Build history of the part. All positions in model axes, mm. Face numbers are marked on the shaded views. A direction names the side the tool comes from. Round coordinates to 2 decimals unless told otherwise and drop trailing zeros. Write each loop counter-clockwise with the first axis right and the second up, starting at its lowest first coordinate (ties: lowest second). Pieces come first, ordered by that corner, then holes. Notation, with made-up numbers: M 86,59 L 124,59 A18 ccw 124,88 Z; hole C 84.5,59.25 d6. An arc over 180 degrees is marked long. Use a Markdown table: item, result.
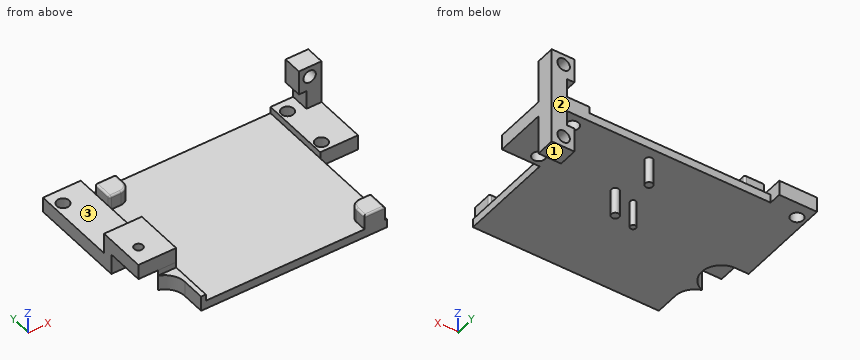
from build123d import *

# Parameters (mm, degrees)
CYLINDER022_R     = 1.15
CYLINDER022_DEPTH = 10
EXTRUDE025_DEPTH  = 1.5
SKETCH022_R       = 0.75
SKETCH022_R_2     = 1
EXTRUDE022_DEPTH  = 8
BOX005_W          = 48
BOX005_H          = 45
BOX005_DEPTH      = 10
SKETCH020_R       = 1.65
EXTRUDE020_DEPTH  = 4
EXTRUDE001_DEPTH  = 4
FILLET003_R       = 0.5
SKETCH021_R       = 1.65
EXTRUDE021_DEPTH  = 5
BOX006_W          = 10
BOX006_H          = 12.95
BOX006_DEPTH      = 4


with BuildPart() as cylinder022:
    # Cylinder022 → Cylinder022 (new body)
    with BuildSketch(Plane(origin=(6.5, 51, 13.03), x_dir=(1, 0, 0), z_dir=(0, 0, 1))):
        Circle(CYLINDER022_R)
    extrude(amount=CYLINDER022_DEPTH)


with BuildPart() as extrude025:
    # Sketch028 → Extrude025 (new body)
    with BuildSketch(Plane.XY):
        with BuildLine():
            Line((8.25, 46.050253), (13, 46.050253))
            Line((13, 46.050253), (13, 59))
            Line((13, 59), (3, 59))
            Line((3, 59), (3, 56.25))
            Line((3, 56.25), (6.5, 56.25))
            ThreePointArc((8.25, 46.050253), (11.674392, 51.887785), (6.5, 56.25))
        make_face()
    extrude(amount=EXTRUDE025_DEPTH)


with BuildPart() as extrude025_1:
    # Extrude025 placement: moved
    add(extrude025.part.moved(Location((0, 0, 17))))


with BuildPart() as extrude022:
    # Sketch022 → Extrude022 (new body)
    with BuildSketch(Plane.XY):
        with Locations((37.45, 61.7)):
            Circle(SKETCH022_R)
        with Locations((42.85, 62.65)):
            Circle(SKETCH022_R_2)
        with Locations((42.85, 75.35)):
            Circle(SKETCH022_R_2)
    extrude(amount=EXTRUDE022_DEPTH)


with BuildPart() as extrude022_1:
    # Extrude022 placement: moved
    add(extrude022.part.moved(Location((0, 0, 6))))


with BuildPart() as obj1:
    # Box005 → Box005 (new body)
    with BuildSketch(Plane(origin=(13, 34, 15.25), x_dir=(1, 0, 0), z_dir=(0, 0, 1))):
        with Locations((24, 22.5)):
            Rectangle(BOX005_W, BOX005_H)
    extrude(amount=BOX005_DEPTH)


with BuildPart() as sensorhold:
    # Sketch020 → Extrude020 (new body)
    with BuildSketch(Plane.XY):
        with BuildLine():
            Line((3, 56.25), (3, 82))
            Line((3, 82), (13, 82))
            Line((13, 82), (13, 78.75))
            Line((13, 78.75), (71, 78.75))
            Line((71, 78.75), (71, 60))
            Line((61, 60), (71, 60))
            Line((61, 34.86), (61, 60))
            Line((11.75, 34.86), (61, 34.86))
            Line((11.75, 34.86), (11.75, 41))
            ThreePointArc((11.75, 41), (10.740672, 44.095028), (8.100781, 46))
            ThreePointArc((8.100781, 46), (11.687123, 51.810093), (6.5, 56.25))
            Line((3, 56.25), (6.5, 56.25))
        make_face()
        with Locations((5.45, 77.95)):
            Circle(SKETCH020_R, mode=Mode.SUBTRACT)
        with Locations((63.15, 62.65)):
            Circle(SKETCH020_R, mode=Mode.SUBTRACT)
        with Locations((63.15, 75.4)):
            Circle(SKETCH020_R, mode=Mode.SUBTRACT)
    extrude(amount=EXTRUDE020_DEPTH)


with BuildPart() as sensorhold_1:
    # Extrude020 placement: moved
    add(sensorhold.part.moved(Location((0, 0, 13))))

    # Cut007: cut obj1
    add(obj1.part, mode=Mode.SUBTRACT)


with BuildPart() as obj2:
    # Sketch001 → Extrude001 (new body)
    with BuildSketch(Plane.XY):
        with BuildLine():
            Line((19.03, 74.44), (19.03, 77.44))
            Line((19.03, 77.44), (13.53, 77.44))
            Line((13.53, 71.94), (13.53, 77.44))
            Line((16.53, 71.94), (13.53, 71.94))
            ThreePointArc((16.53, 71.94), (18.297767, 72.672233), (19.03, 74.44))
        make_face()
        with BuildLine():
            Line((60.53, 34.86), (55.03, 34.86))
            Line((55.03, 34.86), (55.03, 37.86))
            ThreePointArc((57.53, 40.36), (55.762233, 39.627767), (55.03, 37.86))
            Line((60.53, 40.36), (57.53, 40.36))
            Line((60.53, 34.86), (60.53, 40.36))
        make_face()
    extrude(amount=EXTRUDE001_DEPTH)


with BuildPart() as obj2_1:
    # Extrude001 placement: moved
    add(obj2.part.moved(Location((0, 0, 2))))

    # Fillet003
    fillet003_edges = [obj2_1.edges().sort_by_distance(p)[0] for p in [
        (57.78, 34.86, 6),
        (55.03, 36.36, 6),
        (55.762233, 39.627767, 6),
        (60.53, 40.36, 4),
        (59.03, 40.36, 6),
        (60.53, 37.61, 6),
        (18.297767, 72.672233, 6),
        (19.03, 77.44, 4),
        (19.03, 75.94, 6),
        (13.53, 77.44, 4),
        (16.28, 77.44, 6),
        (13.53, 71.94, 4),
        (13.53, 74.69, 6),
        (15.03, 71.94, 6),
    ]]
    fillet(fillet003_edges, radius=FILLET003_R)


with BuildPart() as obj2_2:
    # Fillet003 placement: moved
    add(obj2_1.part.moved(Location((0, 0, 13))))


with BuildPart() as gpshold:
    # Sketch021 → Extrude021 (new body)
    with BuildSketch(Plane.XZ):
        Polygon((65, 28.5), (71, 28.5), (71, 2.5), (65, 2.5), (65, 9), (67, 9), (67, 22), (65, 22), align=None)
        with Locations((67.85, 25.7)):
            Circle(SKETCH021_R, mode=Mode.SUBTRACT)
        with Locations((67.85, 5.4)):
            Circle(SKETCH021_R, mode=Mode.SUBTRACT)
    extrude(amount=EXTRUDE021_DEPTH)


with BuildPart() as gpshold_1:
    # Extrude021 placement: moved
    add(gpshold.part.moved(Location((0, 78.75, 0))))


with BuildPart() as sensorhold003:
    # Box006 → Box006 (new body)
    with BuildSketch(Plane(origin=(3, 46.05, 18.5), x_dir=(1, 0, 0), z_dir=(0, 0, 1))):
        with Locations((5, 6.475)):
            Rectangle(BOX006_W, BOX006_H)
    extrude(amount=BOX006_DEPTH)

    # Fusion025: union Extrude025, Extrude022, SensorHold, obj2, gpsHold
    add(extrude025_1.part)
    add(extrude022_1.part)
    add(sensorhold_1.part)
    add(obj2_2.part)
    add(gpshold_1.part)

    # Cut008: cut Cylinder022
    add(cylinder022.part, mode=Mode.SUBTRACT)


solid = sensorhold003.part
Q1. Drill centre lines: L1, parallel to X at y = 75.4, z = 15.65; L2, parallel to Y at x = 63.15, z = 16.05; L3, parallel to Z at x = 34.5, y = 49. Where is each one in solid material? Low to high.
Response values:
| item | result |
|---|---|
| L1 | x = 3 to 13, 13.53 to 19.03, 61 to 61.5, 64.8 to 71 |
| L2 | y = 60 to 61, 64.3 to 73.75, 77.05 to 78.75 |
| L3 | z = 13 to 15.25 |
Q2. Cut at D-D on z = 14.5. Give the cut face in (x, y), and give its area (3 significant figures).
Response values:
| item | result |
|---|---|
| outline | M 3,56.25 L 6.5,56.25 A5.25 cw 8.1,46 A5.25 cw 11.75,41 L 11.75,34.86 L 61,34.86 L 61,60 L 71,60 L 71,78.75 L 13,78.75 L 13,82 L 3,82 Z; hole C 5.45,77.95 d3.3; hole C 63.15,62.65 d3.3; hole C 63.15,75.4 d3.3 |
| area | 2,570 mm2 |
Q3. Drop flat-ended pins along their axis: P1, Ø1.1, axis at y = 44, z = 14, coming from the +X side; P2, Ø2.5, axis at x = 17, z = 17, coming from the +Y side; P3, Ø23.5, axis at x = 39.5, y = 49, coming from the -Z side; P4, Ø8, axis at x = 43, z = 22.5, coming from the -Y side. Give the stop position or say it passes through.
Response values:
| item | result |
|---|---|
| P1 | stops at x = 61 |
| P2 | stops at y = 77.44 |
| P3 | stops at z = 13 |
| P4 | passes through |
Q4. Cut at C-C on x = 63.15. Give the cut face in (y, z), and give its area (3 significant figures).
Response values:
| item | result |
|---|---|
| outline | M 60,13 L 61,13 L 61,17 L 60,17 Z; M 64.3,13 L 73.75,13 L 73.75,17 L 64.3,17 Z; M 77.05,13 L 78.75,13 L 78.75,17 L 77.05,17 Z |
| area | 48.6 mm2 |
Q5. Which spindle directions (+Z, -Z, +X, -X, +Y, -Y) get a long thin tool onto all of the face, cutting with end or side? Do the marked faces 1, 2 and 3. Say none if no direction does.
Response values:
| item | result |
|---|---|
| face 1 | -Z, +X, -X, +Y, -Y |
| face 2 | +Z, -Z, +X, +Y |
| face 3 | +Z, -X, +Y |
Q6. Cut at B-B on y = 51. Give the cut face in (x, z), and give its area (3 significant figures).
Response values:
| item | result |
|---|---|
| outline | M 3,18.5 L 5.35,18.5 L 5.35,22.5 L 3,22.5 Z; M 7.65,18.5 L 11.75,18.5 L 11.75,13 L 61,13 L 61,15.25 L 13,15.25 L 13,22.5 L 7.65,22.5 Z |
| area | 146 mm2 |
Q7. Cut at A-A on z = 20.5. Give the cut face in (x, y).
Response values:
| item | result |
|---|---|
| outline | M 3,46.05 L 13,46.05 L 13,59 L 3,59 Z; M 67,73.75 L 71,73.75 L 71,78.75 L 67,78.75 Z; hole C 6.5,51 d2.3 |
